The model under review builds one solid part; all positions refer to its coordinate system, in mm. A direction names the side the tool comes from. Coordinates: 2 decimals unless noted, no trailing zeros. Order: outer loops, then holes, each group sorted by start corner. A loop starts at its lowest first (then second) coordinate and runs counter-clockwise, first axis right, second up. Notation, with made-up numbers: (-10.5, -20) -> (35.5, -20) arc R30 cw to (35.5, 17) -> close; hole circle Ø7 at (-18, 87). An arc over 180 degrees is marked (long way). Use one line per item in the form item = value.
from build123d import *

# Parameters (mm, degrees)
F0_W     = 25.4
F0_H     = 25.4
F1_DEPTH = 250
F2_T     = -2
F3_R     = 4.5
F4_DEPTH = 1.6
F5_R     = 4.5
F6_DEPTH = 1.6


with BuildPart() as f1:
    # F0 (on Right) → F1 (new body, symmetric)
    with BuildSketch(Plane.YZ):
        Rectangle(F0_W, F0_H)
    extrude(amount=F1_DEPTH, both=True)

    # F2
    f2_openings = [f1.faces().sort_by_distance(p)[0] for p in [
        (250, 0, 0),
        (-250, 0, 0),
    ]]
    offset(amount=F2_T, openings=f2_openings)

    # F3 (on face) → F4 (join)
    with BuildSketch(Plane.YZ.offset(250)):
        with BuildLine():
            ThreePointArc((42.7, 10.7), (42.114214, 12.114214), (40.7, 12.7))
            Line((40.7, 12.7), (-40.7, 12.7))
            ThreePointArc((-40.7, 12.7), (-42.114214, 12.114214), (-42.7, 10.7))
            Line((-42.7, 10.7), (-42.7, -10.7))
            ThreePointArc((-42.7, -10.7), (-42.114214, -12.114214), (-40.7, -12.7))
            Line((-40.7, -12.7), (40.7, -12.7))
            ThreePointArc((40.7, -12.7), (42.114214, -12.114214), (42.7, -10.7))
            Line((42.7, -10.7), (42.7, 10.7))
        make_face()
        with Locations((-27.7, 0)):
            Circle(F3_R, mode=Mode.SUBTRACT)
        with Locations((27.7, 0)):
            Circle(F3_R, mode=Mode.SUBTRACT)
    extrude(amount=F4_DEPTH)

    # F5 (on face) → F6 (join)
    with BuildSketch(Plane(origin=(-250, 0, 0), x_dir=(0, -1, 0), z_dir=(-1, 0, 0))):
        with BuildLine():
            Line((-12.7, 12.7), (-40.7, 12.7))
            ThreePointArc((-40.7, 12.7), (-42.114214, 12.114214), (-42.7, 10.7))
            Line((-42.7, 10.7), (-42.7, -10.7))
            ThreePointArc((-42.7, -10.7), (-42.114214, -12.114214), (-40.7, -12.7))
            Line((-40.7, -12.7), (-12.7, -12.7))
            Line((-12.7, -12.7), (-12.7, 12.7))
        make_face()
        with Locations((-27.7, 0)):
            Circle(F5_R, mode=Mode.SUBTRACT)
        with BuildLine():
            Line((12.7, 12.7), (-12.7, 12.7))
            Line((-12.7, 12.7), (-12.7, -12.7))
            Line((-12.7, -12.7), (12.7, -12.7))
            Line((12.7, -12.7), (40.7, -12.7))
            ThreePointArc((40.7, -12.7), (42.114214, -12.114214), (42.7, -10.7))
            Line((42.7, -10.7), (42.7, 10.7))
            ThreePointArc((42.7, 10.7), (42.114214, 12.114214), (40.7, 12.7))
            Line((40.7, 12.7), (12.7, 12.7))
        make_face()
        with Locations((27.7, 0)):
            Circle(F5_R, mode=Mode.SUBTRACT)
    extrude(amount=F6_DEPTH)


solid = f1.part
Item 1: Tool access review of faces 1 (the face through (-250, 28, 6)), 2 (the face through (4, 0, 10.7)), 3 (the face through (250, -28, 6)), 4 (the face through (1, 6, -12.7)): name each direction out of +Z, -Z, +X, -X, +Y, -Y from which nothing blocks a thin tool from reaching the whole face with its end or side.
Results found:
face_1 = +Z, -Z, +Y
face_2 = none
face_3 = +Z, -Z, -Y
face_4 = -Z, +X, -X, +Y, -Y
Item 2: Draft analysis for pull direction Y (two halves, no side actions). For faces 5 (the face through (4, -12.7, 0)), 6 (the face through (4, -10.7, 0)), 7 (the face through (1, -6, 12.7)), state which applies: released by +Y, released by -Y, zero draft, split by the parting line, or undercut.
Results found:
face_5 = released by -Y
face_6 = undercut
face_7 = zero draft
Item 3: We need section A-A (z = 0). State how many separate pieces and enclosed holes the cut face has, plus the area to 3 significant figures.
Results found:
separate_pieces = 5
enclosed_holes = 1
area = 2,220 mm²
Item 4: We need section C-C (y = -27.7). Write out the cut boundary in (x, z).
Results found:
outline = (-251.6, -12.7) -> (-250, -12.7) -> (-250, -4.5) -> (-251.6, -4.5) -> close; (-251.6, 4.5) -> (-250, 4.5) -> (-250, 12.7) -> (-251.6, 12.7) -> close; (250, -12.7) -> (251.6, -12.7) -> (251.6, -4.5) -> (250, -4.5) -> close; (250, 4.5) -> (251.6, 4.5) -> (251.6, 12.7) -> (250, 12.7) -> close
Item 5: We need section D-D (x = 153.5). Write out the cut boundary in (y, z).
Results found:
outline = (-12.7, -12.7) -> (12.7, -12.7) -> (12.7, 12.7) -> (-12.7, 12.7) -> close; hole (-10.7, -10.7) -> (10.7, -10.7) -> (10.7, 10.7) -> (-10.7, 10.7) -> close
Item 6: To check wall thickness, follow L1, parallel to Y at x = -5, z = -9.5; L2, parallel to X at y = -22.5, z = 2.25; L3, parallel to Z at x = 250.85, y = -27.7. State the ranges of each line that lie inside material, in increasing order. Write a range as from..to.
Results found:
L1 = -12.7..-10.7, 10.7..12.7
L2 = -251.6..-250, 250..251.6
L3 = -12.7..-4.5, 4.5..12.7
Item 7: Clearance check with flat-ended pins moving along their axes: pin 1 (3 mm diameter, centred on x = 169, z = -7.5, fed in from +Y); pin 2 (10.5 mm diameter, centred on x = 13.5, z = -1, fed in from -Y). State where each tip first meets the part, or that it passes through.
Results found:
pin_1 = 12.7
pin_2 = -12.7
Item 8: We need section B-B (y = 5). Write out the cut boundary in (x, z).
Results found:
outline = (-251.6, -12.7) -> (251.6, -12.7) -> (251.6, 12.7) -> (-251.6, 12.7) -> close; hole (-250, -10.7) -> (250, -10.7) -> (250, 10.7) -> (-250, 10.7) -> close
